Autodesk Inventor part; units mm, degrees
ref_plane "YZ Plane" through (0, 0, 0) normal (1, 0, 0) x (0, 1, 0)
ref_plane "XZ Plane" through (0, 0, 0) normal (0, 1, 0) x (-1, 0, 0)
ref_plane "XY Plane" through (0, 0, 0) normal (0, 0, 1) x (1, 0, 0)
sketch "Sketch1" plane through (0, 0, 0) normal (0, 0, 1) x (1, 0, 0)
  line L0 (-40, -40) -> (40, -40)
  line L1 (40, -40) -> (40, 40)
  line L2 (40, 40) -> (-40, 40)
  line L3 (-40, 40) -> (-40, -40)
  line L4 (-40, -40) -> (40, 40) construction
  line L5 (40, -40) -> (-40, 40) construction
  point P0 (0, 0)
  dimension "d0" = 80
  dimension "d1" = 80
extrude "Extrusion1" add sketch "Sketch1" along normal blind 6
sketch "Sketch2" plane through (0, 0, 0) normal (0, 0, -1) x (-1, 0, 0)
  arc A0 (37, -21.1) -> (40, -18.1) centre (37, -18.1) ccw
  line L0 (37, -21.1) -> (-37, -21.1)
  arc A1 (-40, -18.1) -> (-37, -21.1) centre (-37, -18.1) ccw
  line L1 (-40, -14.1) -> (-40, -18.1)
  arc A2 (-37, -11.1) -> (-40, -14.1) centre (-37, -14.1) ccw
  line L2 (-23, -11.1) -> (-37, -11.1)
  arc A3 (-23, -11.1) -> (-20, -8.1) centre (-23, -8.1) ccw
  line L3 (-20, -8.1) -> (-20, 37)
  arc A4 (-17, 40) -> (-20, 37) centre (-17, 37) ccw
  line L4 (17, 40) -> (-17, 40)
  arc A5 (20, 37) -> (17, 40) centre (17, 37) ccw
  line L5 (20, 37) -> (20, -8.1)
  arc A6 (20, -8.1) -> (23, -11.1) centre (23, -8.1) ccw
  line L6 (37, -11.1) -> (23, -11.1)
  arc A7 (40, -14.1) -> (37, -11.1) centre (37, -14.1) ccw
  line L7 (40, -14.1) -> (40, -18.1)
  circle A8 centre (15, 3.9) radius 2
  circle A9 centre (-15, 3.9) radius 2
  circle A10 centre (15, 23.9) radius 2
  circle A11 centre (-15, 23.9) radius 2
  line L8 (12.1, 32) -> (12.1, -13.1)
  line L9 (-12.1, 32) -> (12.1, 32)
  line L10 (-12.1, -13.1) -> (-12.1, 32)
  line L11 (12.1, -13.1) -> (-12.1, -13.1)
  circle A12 centre (0, -1.1) radius 7.5
  line L12 (-40, -40) -> (40, -40)
  line L13 (40, -40) -> (40, 40)
  line L14 (40, 40) -> (-40, 40)
  line L15 (-40, 40) -> (-40, -40)
  line L16 (-40, -40) -> (40, 40) construction
  line L17 (40, -40) -> (-40, 40) construction
  line L18 (-40, 40) -> (40, 40)
  line L19 (40, 40) -> (40, -40)
  line L20 (-40, -40) -> (-40, 40)
  line L21 (40, -40) -> (-40, -40)
  point P0 (0, 0)
  point P1 (0, 0)
  point P2 (-40, -18.1)
extrude "Extrusion2" cut sketch "Sketch2" against normal blind 6 contours A0 L13 L12 L15 A1 L0 | A7 L6 A6 L5 A5 L14 L13 | L15 L14 A4 L3 A3 L2 A2 | A8 | A9 | A10 | A11 | A12
sketch "Sketch3" plane through (0, 0, 0) normal (0, 0, -1) x (-1, 0, 0)
  arc A0 (37, -21.1) -> (40, -18.1) centre (37, -18.1) ccw
  line L0 (37, -21.1) -> (-37, -21.1)
  arc A1 (-40, -18.1) -> (-37, -21.1) centre (-37, -18.1) ccw
  line L1 (-40, -14.1) -> (-40, -18.1)
  arc A2 (-37, -11.1) -> (-40, -14.1) centre (-37, -14.1) ccw
  line L2 (-23, -11.1) -> (-37, -11.1)
  arc A3 (-23, -11.1) -> (-20, -8.1) centre (-23, -8.1) ccw
  line L3 (-20, -8.1) -> (-20, 37)
  arc A4 (-17, 40) -> (-20, 37) centre (-17, 37) ccw
  line L4 (17, 40) -> (-17, 40)
  arc A5 (20, 37) -> (17, 40) centre (17, 37) ccw
  line L5 (20, 37) -> (20, -8.1)
  arc A6 (20, -8.1) -> (23, -11.1) centre (23, -8.1) ccw
  line L6 (37, -11.1) -> (23, -11.1)
  arc A7 (40, -14.1) -> (37, -11.1) centre (37, -14.1) ccw
  line L7 (40, -14.1) -> (40, -18.1)
  circle A8 centre (15, 3.9) radius 2
  circle A9 centre (-15, 3.9) radius 2
  circle A10 centre (15, 23.9) radius 2
  circle A11 centre (-15, 23.9) radius 2
  line L8 (12.1, 32) -> (12.1, -13.1)
  line L9 (-12.1, 32) -> (12.1, 32)
  line L10 (-12.1, -13.1) -> (-12.1, 32)
  line L11 (12.1, -13.1) -> (-12.1, -13.1)
  point P0 (0, 0)
extrude "Extrusion3" add sketch "Sketch3" along normal blind 5
sketch "Sketch4" plane through (0, 0, 6) normal (0, 0, 1) x (1, 0, 0)
  circle A0 centre (0, -1.1) radius 7.5
  circle A1 centre (0, -1.1) radius 11
  point P0 (0, 0)
  dimension "d8" = 22
extrude "Extrusion4" cut sketch "Sketch4" against normal through all
fillet "Fillet1" radius 3 16 edges at (-19.1213, 39.1213, 6) (-20, 14.45, 6) (-20.8787, -10.2213, 6) (-30, -11.1, 6) (-39.1213, -11.9787, 6) (-40, -16.1, 6) (-39.1213, -20.2213, 6) (0, -21.1, 6) (39.1213, -20.2213, 6) (40, -16.1, 6) (39.1213, -11.9787, 6) (30, -11.1, 6) (20.8787, -10.2213, 6) (20, 14.45, 6) (19.1213, 39.1213, 6) (0, 40, 6)
properties part number "stopper_motor_bracket_cover"
Geometry check sheet. Reference: the model listing, model coordinates, mm. A direction names the side the tool comes from. Coordinates: 2 decimals unless noted, no trailing zeros. Write each loop counter-clockwise with the first axis right and the second up, starting at its lowest first coordinate (ties: lowest second). Pieces come first, ordered by that corner, then holes. Notation, with made-up numbers: (66, 35) -> (83, 35) arc R5 ccw to (83, 42) -> close; hole circle Ø11 at (18.5, -15). An arc over 180 degrees is marked (long way). Use CSV: the item, a comma, the result in double quotes. Start each with the question number.
Item 1: Cross-section at B-B, the plane y = -1.1. Record the cut outline in (x, z), plus the area to 3 significant figures.
Item 2: Cross-section at A-A, the plane x = 0. Record the cut outline in (y, z), plus the area to 3 significant figures.
Item 3: Mould release check, pull along Y, two halves, no side actions. Record for faces 1 (the flat face through (-20, 15, -1)), 2 (the cylindrical face through (-13.4, 25.1, 0.6)), 3 (the flat face through (0, -13.1, -2)), 4 (the flat face through (0, 40, -1)): released by +Y, released by -Y, zero draft, split by the parting line, or undercut.
Item 4: Cross-section at D-D, the plane y = 23.9. State how many separate pieces and enclosed holes the cut face has, plus the area to 3 significant figures.
Item 5: Set-up check for faces 5 (the cylindrical face through (-29.9, -11.96, 5.1)), 6 (the flat face through (0, 32, -2)), 7 (the flat face through (30, -11.1, -1)), 8 (the cylindrical face through (-39.14, -20.2, -0.94)): record each of +Z, -Z, +X, -X, +Y, -Y from which the full face is reachable in a straight line by a thin tool's end or side.
Item 6: Cross-section at C-C, the plane z = 1. Record the cut outline in (x, y).
Item 7: Thickness scan on line 1 (Y direction, x = 15, z = -1.75); line 2 (X direction, y = -2.5, z = -2); line 3 (Y direction, x = 35, z = 2). Record the ranges inside material, lowest first.
Item 8: Depth check by flat-ended pin: pin 1 Ø5 at (x, y) = (-9, -2.5) entering from -Z; pin 2 Ø5.5 at (y, z) = (12, -1.5) entering from +X; pin 3 Ø2.5 at (x, z) = (-32, 0.5) entering from +Y. Enter the tip coordinate at first touch or a pass-through.
Answers:
1,outline,"(-20, -5) -> (-12.1, -5) -> (-12.1, 0) -> (-11, 0) -> (-11, 6) -> (-17, 6) arc R3 ccw to (-20, 3) -> close; (11, 0) -> (12.1, 0) -> (12.1, -5) -> (20, -5) -> (20, 3) arc R3 ccw to (17, 6) -> (11, 6) -> close"
1,area,"183 mm^2"
2,outline,"(-21.1, -5) -> (-13.1, -5) -> (-13.1, 0) -> (-12.1, 0) -> (-12.1, 6) -> (-18.1, 6) arc R3 ccw to (-21.1, 3) -> close; (9.9, 0) -> (32, 0) -> (32, -5) -> (40, -5) -> (40, 3) arc R3 ccw to (37, 6) -> (9.9, 6) -> close"
2,area,"311 mm^2"
3,face 1,"zero draft"
3,face 2,"undercut"
3,face 3,"undercut"
3,face 4,"released by +Y"
4,separate pieces,"3"
4,enclosed holes,"0"
4,area,"227 mm^2"
5,face 5,"+Z, -X, +Y"
5,face 6,"-Z"
5,face 7,"+Z, -Z, +X, +Y"
5,face 8,"+Z, -Z, -X, -Y"
6,outline,"(-40, -18.1) arc R3 ccw to (-37, -21.1) -> (37, -21.1) arc R3 ccw to (40, -18.1) -> (40, -14.1) arc R3 ccw to (37, -11.1) -> (23, -11.1) arc R3 cw to (20, -8.1) -> (20, 37) arc R3 ccw to (17, 40) -> (-17, 40) arc R3 ccw to (-20, 37) -> (-20, -8.1) arc R3 cw to (-23, -11.1) -> (-37, -11.1) arc R3 ccw to (-40, -14.1) -> close; hole circle Ø4 at (-15, 3.9); hole circle Ø4 at (-15, 23.9); hole circle Ø22 at (0, -1.1); hole circle Ø4 at (15, 3.9); hole circle Ø4 at (15, 23.9)"
7,line 1,"-21.1 to 1.9, 5.9 to 21.9, 25.9 to 40"
7,line 2,"-20 to -12.1, 12.1 to 20"
7,line 3,"-21.1 to -11.1"
8,pin 1,"z = 0"
8,pin 2,"x = 20"
8,pin 3,"y = -11.1"
